from build123d import *

# Parameters (mm, degrees)
EXTRUDE2_DEPTH = 115.5


with BuildPart() as part:
    # Sketch1 → Extrude2 (new body)
    with BuildSketch(Plane.XY.offset(-35.173777659)):
        Polygon((85.961408719, 43.751957214), (94.761408719, 43.751957214), (94.761408719, 51.676244301), (99.761408719, 51.676244301), (99.761408719, 27.051957214), (94.761408719, 27.051957214), (94.761408719, 36.351957214), (85.961408719, 36.351957214), align=None)
    extrude(amount=-EXTRUDE2_DEPTH)


solid = part.part
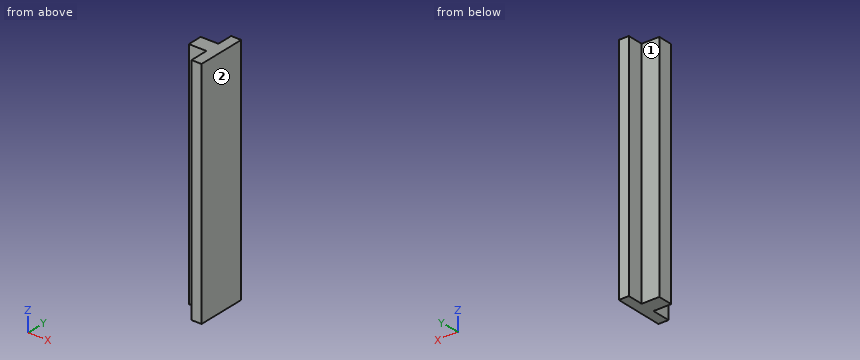
Build history of the part. All positions in model axes, mm. Face numbers are marked on the shaded views. A direction names the side the tool comes from. Give positions to 0.01 mm unless a question says otherwise; leave off trailing zeros. Write each loop counter-clockwise with the first axis right and the second up, starting at its lowest first coordinate (ties: lowest second). Pieces come first, ordered by that corner, then holes. Notation, with made-up numbers: (82, 14) - (123, 14) arc R19 cw to (123, 40) - close; hole circle Ø2 at (23, 24.25). An arc over 180 degrees is marked (long way). Use one line per item in the form item = value. Start each with the question number.
1. Band-saw the part on B-B on x = 89.75. Write the cut outline in (y, z).
2. Band-saw the part on C-C on y = 45.5. Write the cut outline in (x, z).
3. Band-saw the part on A-A on z = -78. Write the cut outline in (x, y).
4. Probe line 1 (Y direction, x = 89, z = -136.5); line 2 (X direction, y = 49.75, z = -72.5). List the from-to ranges inside material, lowest first. Write a range as [from, to].
5. 3-axis set-ups, long thin cutter, end or side, ignore diameter. For the marked faces 1 and 2: which of +Z, -Z, +X, -X, +Y, -Y reach the whole face in a straight line?
6. Drop flat-ended pins along their axis: pin 1 Ø6 at (x, z) = (89.5, -119) entering from +Y; pin 2 Ø7.5 at (y, z) = (30.5, -96.5) entering from -X; pin 3 Ø4.5 at (x, z) = (90.5, -99) entering from -Y. Give the stop position or say it passes through.
Conclusion:
q1.outline = (36.35, -150.67) - (43.75, -150.67) - (43.75, -35.17) - (36.35, -35.17) - close
q2.outline = (94.76, -150.67) - (99.76, -150.67) - (99.76, -35.17) - (94.76, -35.17) - close
q3.outline = (85.96, 36.35) - (94.76, 36.35) - (94.76, 27.05) - (99.76, 27.05) - (99.76, 51.68) - (94.76, 51.68) - (94.76, 43.75) - (85.96, 43.75) - close
q4.line_1 = [36.35, 43.75]
q4.line_2 = [94.76, 99.76]
q5.face_1 = +Z, -Z, -X, +Y
q5.face_2 = +Z, -Z, +X, +Y, -Y
q6.pin_1 = 43.75
q6.pin_2 = 94.76
q6.pin_3 = 36.35
